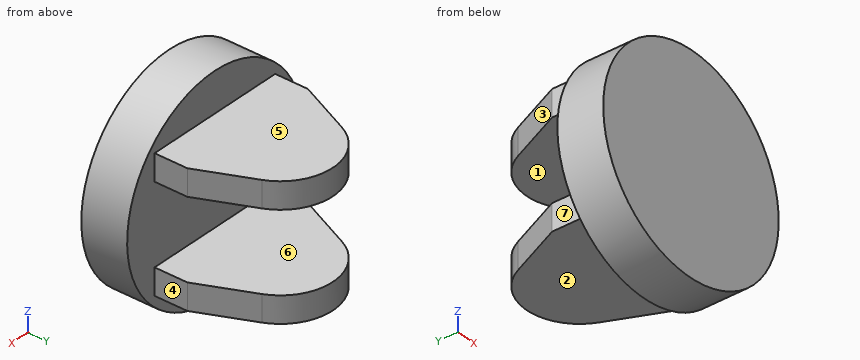
```python
from build123d import *

# Parameters (mm, degrees)
CROQUIS1_W              = 15
CROQUIS1_H              = 50
CROQUIS1_W_2            = 50
CROQUIS1_H_2            = 115
SALIENTE_EXTRUIR1_DEPTH = 250
CROQUIS2_R              = 80
SALIENTE_EXTRUIR2_DEPTH = 35
SALIENTE_EXTRUIR3_DEPTH = 50
CROQUIS4_W              = 60
CROQUIS4_H              = 90
CORTAR_EXTRUIR1_DEPTH   = 407.509532484
CROQUIS5_R              = 80
CORTAR_EXTRUIR2_DEPTH   = 283.710098865


with BuildPart() as part:
    # Croquis1 → Saliente-Extruir1 (new body)
    with BuildSketch(Plane(origin=(0, 0, 0), x_dir=(1, 0, 0), z_dir=(0, 1, 0))):
        with Locations((-32.5, 0)):
            Rectangle(CROQUIS1_W, CROQUIS1_H)
        Rectangle(CROQUIS1_W_2, CROQUIS1_H_2)
    extrude(amount=SALIENTE_EXTRUIR1_DEPTH)

    # Croquis2 → Saliente-Extruir2 (add)
    with BuildSketch(Plane(origin=(0, 250, 0), x_dir=(1, 0, 0), z_dir=(0, 1, 0))):
        with Locations(Location((-25, 0, 0), (0, 0, 270))):
            Circle(CROQUIS2_R)
    extrude(amount=SALIENTE_EXTRUIR2_DEPTH)

    # Croquis3 → Saliente-Extruir3 (add, symmetric)
    with BuildSketch(Plane.XY):
        with BuildLine():
            Line((11.514226217, 351.331297677), (30, 310))
            Line((30, 310), (30, 285))
            Line((30, 285), (-80, 285))
            Line((-80, 285), (-80, 310))
            Line((-80, 310), (-61.514226217, 351.331297677))
            ThreePointArc((-61.514226217, 351.331297677), (-25, 375), (11.514226217, 351.331297677))
        make_face()
    extrude(amount=SALIENTE_EXTRUIR3_DEPTH, both=True)

    # Croquis4 → Cortar-Extruir1 (cut, through all)
    with BuildSketch(Plane(origin=(30, 0, 0), x_dir=(0, 0, -1), z_dir=(1, 0, 0))):
        with Locations((0, 330)):
            Rectangle(CROQUIS4_W, CROQUIS4_H)
    extrude(amount=-CORTAR_EXTRUIR1_DEPTH, mode=Mode.SUBTRACT)

    # Croquis5 → Cortar-Extruir2 (cut, through all)
    with BuildSketch(Plane.XZ.offset(-250)):
        with Locations(Location((-25, 0, 0), (0, 0, 90))):
            Circle(CROQUIS5_R)
    extrude(amount=CORTAR_EXTRUIR2_DEPTH, mode=Mode.SUBTRACT)


solid = part.part
```
CAD build for the part. Positions are in the model's coordinates, mm. Face numbers are marked on the shaded views. A direction names the side the tool comes from. Round coordinates to 2 decimals unless told otherwise and drop trailing zeros. Write each loop counter-clockwise with the first axis right and the second up, starting at its lowest first coordinate (ties: lowest second). Pieces come first, ordered by that corner, then holes. Notation, with made-up numbers: (9, -8) -> (22, -8) arc R28 ccw to (22, 22) -> close; hole circle Ø3 at (45, 63). An arc over 180 degrees is marked (long way). Answer in a Markdown table with one row per item. Add a question column.
Item 1: Saw through at A-A, the plane y = 287.5. Write the cut outline in (x, z).
Item 2: Saw through at B-B, the plane x = -25. Write the cut outline in (y, z), then the cut area to 3 significant figures.
Item 3: Saw through at D-D, the plane y = 346.5. Write the cut outline in (x, z), then the cut area to 3 significant figures.
Item 4: Saw through at C-C, the plane z = -41. Write the cut outline in (x, y).
Item 5: Mould opens along Z. For the marked faces 1, 2 and 3 say: pulls with the +Z half, pulls with the -Z half, needs draft (parallel to the pull), parting line crosses it, or undercut.
Item 6: Drill centre lines: line 1 (Z direction, x = -46, y = 312.5); line 2 (Y direction, x = 8.5, z = 53); line 3 (X direction, y = 307, z = -38). Where is each one in solid material? Low to high. Write a range as from..to.
Item 7: Which spindle directions (+Z, -Z, +X, -X, +Y, -Y) get a long thin tool onto all of the face, cutting with end or side? Do the marked faces 4, 5, 6 and 7. Say none if no direction does.
Item 8: Drop flat-ended pins along their axis: pin 1 Ø22 at (y, z) = (300.5, 44) entering from -X; pin 2 Ø8 at (y, z) = (274.5, -38.5) entering from +X; pin 3 Ø22 at (y, z) = (291.5, -40) entering from -X. Give the stop position or say it passes through.
Findings below:
| question | item | result |
|---|---|---|
| 1 | outline | (-80, -50) -> (30, -50) -> (30, -30) -> (-80, -30) -> close; (-80, 30) -> (30, 30) -> (30, 50) -> (-80, 50) -> close |
| 2 | outline | (250, -80) -> (285, -80) -> (285, -50) -> (375, -50) -> (375, -30) -> (285, -30) -> (285, 30) -> (375, 30) -> (375, 50) -> (285, 50) -> (285, 80) -> (250, 80) -> close |
| 2 | area | 9,200 mm^2 |
| 3 | outline | (-63.68, -50) -> (13.68, -50) -> (13.68, -30) -> (-63.68, -30) -> close; (-63.68, 30) -> (13.68, 30) -> (13.68, 50) -> (-63.68, 50) -> close |
| 3 | area | 3,090 mm^2 |
| 4 | outline | (-93.69, 250) -> (43.69, 250) -> (43.69, 285) -> (30, 285) -> (30, 310) -> (11.51, 351.33) arc R40 ccw to (-61.51, 351.33) -> (-80, 310) -> (-80, 285) -> (-93.69, 285) -> close |
| 5 | face 1 | undercut |
| 5 | face 2 | pulls with the -Z half |
| 5 | face 3 | needs draft |
| 6 | line 1 | z = -50..-30, 30..50 |
| 6 | line 2 | y = 250..285 |
| 6 | line 3 | x = -80..30 |
| 7 | face 4 | +Z, -Z, +X, +Y |
| 7 | face 5 | +Z, +X, -X, +Y |
| 7 | face 6 | +X, -X, +Y |
| 7 | face 7 | +Z, -Z, -X, +Y |
| 8 | pin 1 | stops at x = -80 |
| 8 | pin 2 | stops at x = 47.18 |
| 8 | pin 3 | stops at x = -98.7 |
